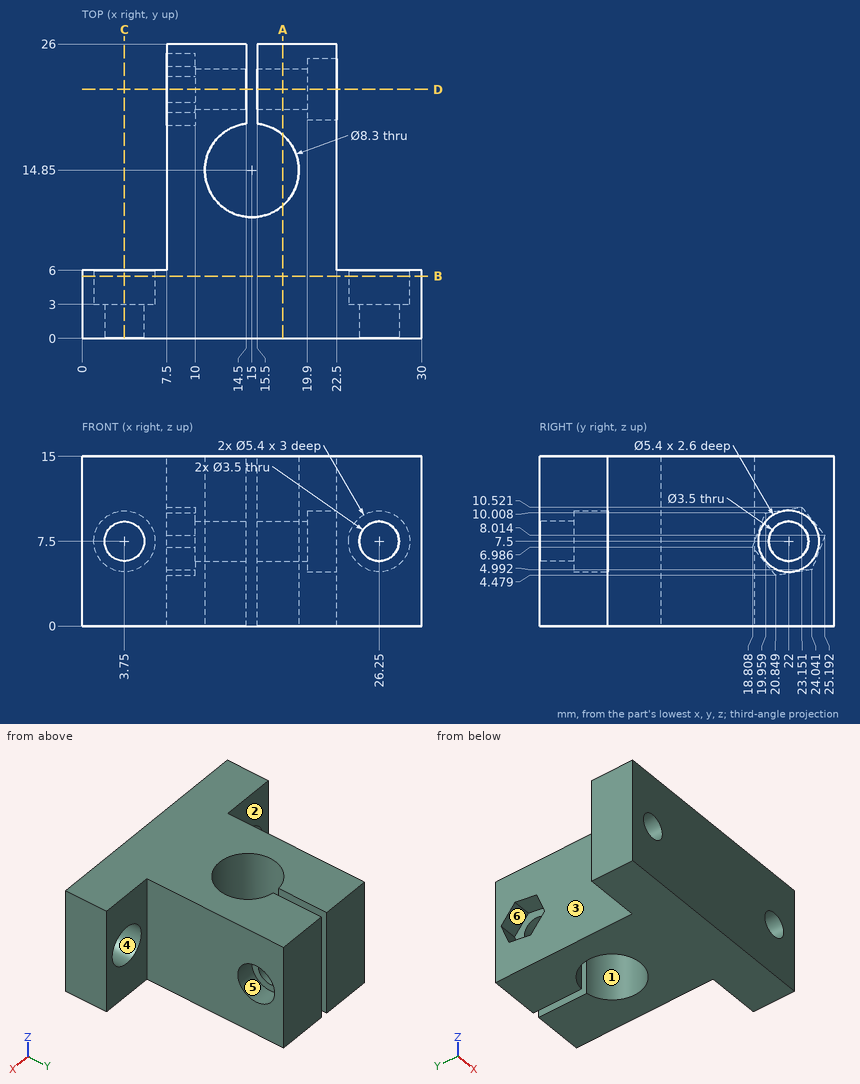
Could you check a few things on this drawing? It's one solid part, dimensions in mm from its lowest x, y, z. A direction names the side the tool comes from. Coordinates: 2 decimals unless noted, no trailing zeros. Order: outer loops, then holes, each group sorted by start corner. A loop starts at its lowest first (then second) coordinate and runs counter-clockwise, first axis right, second up. Notation, with made-up numbers: M 88,-11 L 142,-11 A28 cw 142,23 Z; hole C 34,-27 d1. An arc over 180 degrees is marked long. Answer as a JSON object with one key per item and string values. Group by question number.
(1) Suppose I cut it at B-B, the plane y = 5.5. Please give me the cut outline in (x, z), then the cut area to 3 significant figures.
(2) For pin 1 (1.8 mm diameter, centred on y = 20.5, z = 8, fed in from -X); pin 2 (3 mm diameter, centred on x = 5, z = 10, fed in from +Y); pin 3 (2.5 mm diameter, centred on y = 23, z = 8, fed in from +X); pin 4 (2 mm diameter, centred on y = 22, z = 7.5, fed in from -X), each with a flat end and sliding along its axis, tell me the tip position at first contact or that it passes through.
(3) Which directions (+Z, -Z, +X, -X, +Y, -Y) give clear straight access to the entire face, cutting with the end or side of a thin tool? Please do the marked faces 4, 5 and 6.
(4) If we mould it in two halves opening along X, with no side actions, what happens to the marked faces 1, 2 and 3? For each: released by +X, released by -X, zero draft, split by the parting line, or undercut.
(5) Suppose I cut it at C-C, the plane x = 3.75. Please give me the cut outline in (y, z).
(6) I need wall thicknesses on probe 1 along Z at (x, y) = (13, 22); probe 2 along X at (y, z) = (20.5, 12.25); probe 3 along Z at (x, y) = (21.8, 22). Which ranges of each line are inside material? Lowest first, please.
(7) Suppose I cut it at A-A, the plane x = 17.75. Please give me the cut outline in (y, z), then the cut area to 3 significant figures.
(8) Suppose I cut it at D-D, the plane y = 22. Please give me the cut outline in (x, z).
Values found:
{
 "1": {"outline": "M 0,0 L 30,0 L 30,15 L 0,15 Z; hole C 3.75,7.5 d5.4; hole C 26.25,7.5 d5.4", "area": "404 mm^2"},
 "2": {"pin 1": "stops at x = 10", "pin 2": "stops at y = 6", "pin 3": "stops at x = 19.9", "pin 4": "passes through"},
 "3": {"face 4": "+Y", "face 5": "+X", "face 6": "-X"},
 "4": {"face 1": "undercut", "face 2": "zero draft", "face 3": "released by -X"},
 "5": {"outline": "M 0,0 L 6,0 L 6,4.8 L 3,4.8 L 3,5.75 L 0,5.75 Z; M 0,9.25 L 3,9.25 L 3,10.2 L 6,10.2 L 6,15 L 0,15 Z"},
 "6": {"probe 1": "z = 0 to 5.75, 9.25 to 15", "probe 2": "x = 7.5 to 14.5, 15.5 to 22.5", "probe 3": "z = 0 to 4.8, 10.2 to 15"},
 "7": {"outline": "M 0,0 L 11.74,0 L 11.74,15 L 0,15 Z; M 17.96,0 L 26,0 L 26,15 L 17.96,15 Z; hole C 22,7.5 d3.5", "area": "287 mm^2"},
 "8": {"outline": "M 7.5,0 L 14.5,0 L 14.5,5.75 L 10,5.75 L 10,4.66 L 7.5,4.66 Z; M 7.5,10.34 L 10,10.34 L 10,9.25 L 14.5,9.25 L 14.5,15 L 7.5,15 Z; M 15.5,0 L 22.5,0 L 22.5,4.8 L 19.9,4.8 L 19.9,5.75 L 15.5,5.75 Z; M 15.5,9.25 L 19.9,9.25 L 19.9,10.2 L 22.5,10.2 L 22.5,15 L 15.5,15 Z"}
}
